Verification items for the finished model (mm, model axes). A direction names the side the tool comes from. Give positions to 0.01 mm unless a question says otherwise; leave off trailing zeros. Write each loop counter-clockwise with the first axis right and the second up, starting at its lowest first coordinate (ties: lowest second). Pieces come first, ordered by that corner, then holes. Notation, with made-up numbers: M 71,26 L 129,26 A16 cw 129,41 Z; hole C 40.25,-1.75 d10. An arc over 180 degrees is marked long. Write item = value, one per line.
from build123d import *

# Parameters (mm, degrees)
CIRPATTERN1_COUNT = 12


with BuildPart() as part:
    # Sketch2 → Revolve1 (revolve)
    with BuildSketch(Plane.YZ, mode=Mode.PRIVATE) as revolve1_sk:
        Polygon((-11.743521681, 3.755235238), (-14.803521681, 6.815235238), (-19.967183183, 0.704867009), (-17.743521681, -1.559764762), (-17.743521681, -4.244764762), (1.256478319, -4.244764762), (1.256478319, -1.559764762), (1.256478319, 3.755235238), align=None)
    revolve(revolve1_sk.sketch.rotate(Axis((0, -25.391509901, -9.244764762), (0, 1, 0)), 180), axis=Axis((0, -25.391509901, -9.244764762), (0, 1, 0)))

    # Cut-Sweep1: sweep along a path in Sketch8
    with BuildLine(Plane.YZ) as cut_sweep1_path:
        Line((-28.743521681, -9.244764762), (-15.053364124, 6.955349006))
    # Sketch9 → Cut-Sweep1 (sweep, cut)
    with BuildSketch(Plane.XY.offset(-9.244764762)):
        Polygon((3.464101615, -30.743521681), (0, -24.743521681), (-3.464101615, -30.743521681), align=None)
    cut_sweep1 = sweep(path=cut_sweep1_path.line, mode=Mode.SUBTRACT)

    # CirPattern1: Cut-Sweep1 ×12 about axis
    cirpattern1_axis = Axis((0, 0, -9.244764762), (0, 1, 0))
    for i in range(1, CIRPATTERN1_COUNT):
        add(cut_sweep1.rotate(cirpattern1_axis, i * 360 / CIRPATTERN1_COUNT), mode=Mode.SUBTRACT)


solid = part.part
1) Tool access check on faces 4 (the flat face through (-12, -16.34, -10.25)), 5 (the flat face through (-1.054, -16.427, -21.247)), 6 (the flat face through (12, -16.43, -10.3)), 7 (the flat face through (5, -17.744, -11)). Record the directions out of +Z, -Z, +X, -X, +Y, -Y that give a thin tool (end or side, any length) a straight path to the whole face; none if there is none.
From the geometry:
face_4 = -X, -Y
face_5 = -Z, -Y
face_6 = +X, -Y
face_7 = -Y
2) Cross-section at B-B on y = -12.25. Record the boundary of the cut face in (x, z).
From the geometry:
outline = C 0,-9.24 d27.01; hole C 0,-9.24 d10
3) Cross-section at A-A on y = -7.5. Record the boundary of the cut face in (x, z).
From the geometry:
outline = C 0,-9.24 d26; hole C 0,-9.24 d10
4) Material ranges on probe 1 along Y at (x, z) = (-4, -4); probe 2 along Z at (x, y) = (-2, -4); probe 3 along Z at (x, y) = (9.5, -17.25), recorded low to high. Write a range as from..to.
From the geometry:
probe_1 = -17.74..1.26
probe_2 = -22.09..-13.83, -4.66..3.6
probe_3 = -18.36..-16.38, -13.81..-9.55, -8.94..-4.68, -2.11..-0.13
5) Depth check by flat-ended pin: P1, Ø2, axis at x = 3, y = -7.5, coming from the +Z side; P2, Ø7.5, axis at x = 1, z = -6, coming from the -Y side; P3, Ø5, axis at x = -7, y = -8, coming from the +Z side; P4, Ø6, axis at x = 0, z = -9.24, coming from the +Y side. Enter the tip coordinate at first touch or a pass-through.
From the geometry:
P1 = 3.6
P2 = -17.74
P3 = 2.95
P4 = through
6) Draft check along Z on faces 1 (the flat face through (0, 1.256, -4)), 2 (the conical face through (-9.66, -16.85, 0.38)), 3 (the flat face through (5.13, -16.34, 1.65)). Enter one of: +Z half, -Z half, draft (parallel to the pull), parting line (faces both ways), or undercut.
From the geometry:
face_1 = draft
face_2 = +Z half
face_3 = undercut
